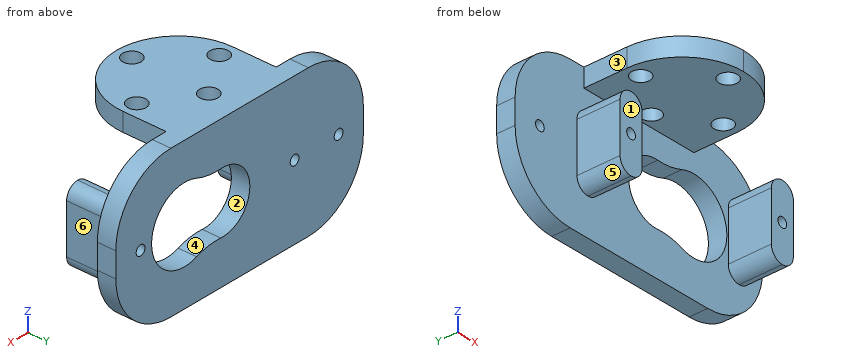
from build123d import *

# Parameters (mm, degrees)
SKETCH1_W           = 45
SKETCH1_H           = 24
BOSS_EXTRUDE1_DEPTH = 3
SKETCH2_R           = 0.8
CUT_EXTRUDE1_DEPTH  = 26.675864153
SKETCH3_W           = 4
SKETCH3_H           = 12
BOSS_EXTRUDE2_DEPTH = 7
SKETCH4_R           = 0.8
CUT_EXTRUDE2_DEPTH  = 5
FILLET1_R           = 2
FILLET2_R           = 10
SKETCH6_W           = 20
SKETCH6_H           = 3
BOSS_EXTRUDE3_DEPTH = 17
FILLET3_R           = 10
SKETCH7_R           = 1.5
CUT_EXTRUDE3_DEPTH  = 3


with BuildPart() as part:
    # Sketch1 → Boss-Extrude1 (new body)
    with BuildSketch(Plane(origin=(0, 0, 0), x_dir=(1, 0, 0), z_dir=(0, 1, 0))):
        Rectangle(SKETCH1_W, SKETCH1_H)
    extrude(amount=BOSS_EXTRUDE1_DEPTH)

    # Sketch2 → Cut-Extrude1 (cut, through all)
    with BuildSketch(Plane(origin=(0, 3, 0), x_dir=(1, 0, 0), z_dir=(0, 1, 0))):
        with Locations(Location((18, 0, 0), (0, 0, 270))):
            Circle(SKETCH2_R)
        with Locations(Location((-10, 0, 0), (0, 0, 270))):
            Circle(SKETCH2_R)
        with Locations(Location((-18, 0, 0), (0, 0, 270))):
            Circle(SKETCH2_R)
        with BuildLine():
            ThreePointArc((7.809591844, -5.585885079), (16, 0), (7.809591844, 5.585885079))
            ThreePointArc((7.809591844, 5.585885079), (5.65712524, 5.008562723), (3.430251149, 4.922276176))
            ThreePointArc((3.430251149, 4.922276176), (-1.864767372, 0), (3.430251149, -4.922276176))
            ThreePointArc((3.430251149, -4.922276176), (5.65712524, -5.008562723), (7.809591844, -5.585885079))
        make_face()
    extrude(amount=-CUT_EXTRUDE1_DEPTH, mode=Mode.SUBTRACT)

    # Sketch3 → Boss-Extrude2 (add)
    with BuildSketch(Plane.XZ):
        with Locations((-9.25, 0)):
            Rectangle(SKETCH3_W, SKETCH3_H)
        with Locations((18.25, 0)):
            Rectangle(SKETCH3_W, SKETCH3_H)
    extrude(amount=BOSS_EXTRUDE2_DEPTH)

    # Sketch4 → Cut-Extrude2 (cut)
    with BuildSketch(Plane.XZ.offset(7)):
        with Locations(Location((18.25, 0, 0), (0, 0, 270))):
            Circle(SKETCH4_R)
        with Locations(Location((-9.25, 0, 0), (0, 0, 270))):
            Circle(SKETCH4_R)
    extrude(amount=-CUT_EXTRUDE2_DEPTH, mode=Mode.SUBTRACT)

    # Fillet1
    fillet1_edges = [part.edges().sort_by_distance(p)[0] for p in [
        (16.25, -3.5, -6),
        (-11.25, -3.5, -6),
        (-7.25, -3.5, -6),
        (20.25, -3.5, -6),
        (-11.25, -3.5, 6),
        (-7.25, -3.5, 6),
        (16.25, -3.5, 6),
        (20.25, -3.5, 6),
    ]]
    fillet(fillet1_edges, radius=FILLET1_R - 0.0001)  # a hair under: the kernel refuses the full size

    # Fillet2
    fillet2_edges = [part.edges().sort_by_distance(p)[0] for p in [
        (-22.5, 1.5, -12),
        (22.5, 1.5, -12),
        (22.5, 1.5, 12),
        (-22.5, 1.5, 12),
    ]]
    fillet(fillet2_edges, radius=FILLET2_R)

    # Sketch6 → Boss-Extrude3 (add)
    with BuildSketch(Plane.XZ):
        with Locations((0, 10.5)):
            Rectangle(SKETCH6_W, SKETCH6_H)
    extrude(amount=BOSS_EXTRUDE3_DEPTH)

    # Fillet3
    fillet3_edges = [part.edges().sort_by_distance(p)[0] for p in [
        (-10, -17, 10.5),
        (10, -17, 10.5),
    ]]
    fillet(fillet3_edges, radius=FILLET3_R - 0.0001)  # a hair under: the kernel refuses the full size

    # Sketch7 → Cut-Extrude3 (cut)
    with BuildSketch(Plane.XY.offset(12)):
        with Locations((0, -14.5)):
            Circle(SKETCH7_R)
        with Locations((0, -2)):
            Circle(SKETCH7_R)
        with Locations((7.5, -7)):
            Circle(SKETCH7_R)
        with Locations((-7.5, -7)):
            Circle(SKETCH7_R)
    extrude(amount=-CUT_EXTRUDE3_DEPTH, mode=Mode.SUBTRACT)


solid = part.part
Geometry: final body of the model. Coordinates: model frame, mm. Face numbers are marked on the shaded views. A direction names the side the tool comes from. Round coordinates to 2 decimals unless told otherwise and drop trailing zeros. Order: outer loops, then holes, each group sorted by start corner. A loop starts at its lowest first (then second) coordinate and runs counter-clockwise, first axis right, second up. Notation, with made-up numbers: (37, 68.5) - (44, 68.5) arc R20 cw to (44, 98.5) - close; hole circle Ø11 at (67.25, 49.25). An arc over 180 degrees is marked (long way). Write each question's results on one line, items separated by ' | '.
Item 1: Mould query, pull axis X, two halves, no side actions, for the marked faces 1, 2 and 3. Classes: pulls with the +X half, pulls with the -X half, needs draft (parallel to the pull), parting line crosses it, or undercut.
Completed:
face 1: needs draft | face 2: undercut | face 3: pulls with the -X half
Item 2: Section B-B, the plane y = -7.5. Return the cut outline in (x, z), and give its area (3 significant figures).
Completed:
outline: (-9.99, 9) - (-8.91, 9) - (-8.91, 12) - (-9.99, 12) - close; (-6.09, 9) - (6.09, 9) - (6.09, 12) - (-6.09, 12) - close; (8.91, 9) - (9.99, 9) - (9.99, 12) - (8.91, 12) - close | area: 43.0 mm^2
Item 3: Section C-C, the plane z = -1.25. Return the cut outline in (x, y).
Completed:
outline: (-22.5, 0) - (-11.25, 0) - (-11.25, -7) - (-7.25, -7) - (-7.25, 0) - (-1.7, 0) - (-1.7, 3) - (-22.5, 3) - close; (15.87, 0) - (16.25, 0) - (16.25, -7) - (20.25, -7) - (20.25, 0) - (22.5, 0) - (22.5, 3) - (15.87, 3) - close
Item 4: Reachability of the marked faces 4, 5 and 6 from +Z, -Z, +X, -X, +Y, -Y: full face, straight path, thin tool, end or side. Return the list, or none.
Completed:
face 4: +Y, -Y | face 5: -Z, -X, -Y | face 6: +Z, -Z, +X, -Y
Item 5: Material intervals for line 1 along Y through (x, z) = (0, 10.1); line 2 along X through (y, z) = (-3.2, 0); line 3 along Z through (x, y) = (4, 0.75), sorted ascending. Write a range as [from, to].
Completed:
line 1: [-17, -16], [-13, -3.5], [-0.5, 3] | line 2: [-11.25, -10.05], [-8.45, -7.25], [16.25, 17.45], [19.05, 20.25] | line 3: [-12, -4.9], [4.9, 12]
Item 6: Section A-A, the plane y = -14.5. Return the cut outline in (x, z), and give its area (3 significant figures).
Completed:
outline: (-6.61, 9) - (-1.5, 9) - (-1.5, 12) - (-6.61, 12) - close; (1.5, 9) - (6.61, 9) - (6.61, 12) - (1.5, 12) - close | area: 30.7 mm^2
Item 7: Section D-D, the plane x = -18. Return the cut outline in (y, z), and give its area (3 significant figures).
Completed:
outline: (0, -10.35) - (3, -10.35) - (3, -0.8) - (0, -0.8) - close; (0, 0.8) - (3, 0.8) - (3, 10.35) - (0, 10.35) - close | area: 57.3 mm^2
Item 8: First-contact query: pin 1 Ø3.5 at (y, z) = (-3, 10.5) entering from -X; pin 2 Ø5.5 at (y, z) = (-3, -1) entering from +X; pin 3 Ø10 at (x, y) = (-16.5, -12) entering from -Z; pin 4 Ø1 at (x, y) = (-1, -12) entering from -Z. Flat tips, straight axial feed; report the tip coordinate or a pass-through.
Completed:
pin 1: x = -10 | pin 2: x = 20.25 | pin 3: through | pin 4: z = 9
